Check sheet for the modelled part. Datum: model origin and axes. Units: mm. A direction names the side the tool comes from. Coordinates: 2 decimals unless noted, no trailing zeros. Loops run counter-clockwise (first coordinate to the right, second up) from the corner with the lowest first, then second, coordinate; pieces in that order, holes last. Notation, with made-up numbers: M -28,-23.75 L -21,-23.75 A34 cw -21,11.25 Z; hole C -14,-15.5 d8. An arc over 180 degrees is marked long. Return JSON: item names as keys, results as strings.
from build123d import *

# Parameters (mm, degrees)
SKETCH1_R           = 9.5
SKETCH1_R_2         = 3
BOSS_EXTRUDE1_DEPTH = 6


with BuildPart() as part:
    # Sketch1 → Boss-Extrude1 (new body)
    with BuildSketch(Plane(origin=(0, 0, 0), x_dir=(1, 0, 0), z_dir=(0, 1, 0))):
        Circle(SKETCH1_R)
        Circle(SKETCH1_R_2, mode=Mode.SUBTRACT)
    extrude(amount=BOSS_EXTRUDE1_DEPTH)

    # Sketch2 → Cut-Revolve1 (revolve, cut)
    with BuildSketch(Plane.XY):
        Polygon((-3.75, 6), (-4.75, 5.5), (-7.75, 5.5), (-8.75, 6), align=None)
        Polygon((-8.75, 0), (-3.75, 0), (-4.75, 0.5), (-7.75, 0.5), align=None)
    revolve(axis=Axis((0, 6, 0), (0, -1, 0)), mode=Mode.SUBTRACT)


solid = part.part
1) Section check A-A on x = 0. Record the cut outline in (y, z).
Answers:
{"outline": "M 0,-9.5 L 6,-9.5 L 6,-8.75 L 5.5,-7.75 L 5.5,-4.75 L 6,-3.75 L 6,-3 L 0,-3 L 0,-3.75 L 0.5,-4.75 L 0.5,-7.75 L 0,-8.75 Z; M 0,3 L 6,3 L 6,3.75 L 5.5,4.75 L 5.5,7.75 L 6,8.75 L 6,9.5 L 0,9.5 L 0,8.75 L 0.5,7.75 L 0.5,4.75 L 0,3.75 Z"}
2) Draft check along X on faces 4 (the face through (4.38, 2.96, 8.43)), 5 (the face through (-3, 3, 0)), 6 (the face through (1, 0, -3)). Enter one of: +X half, -X half, draft (parallel to the pull), parting line (faces both ways), or undercut.
Answers:
{"face 4": "parting line", "face 5": "undercut", "face 6": "draft"}
3) Scan lines: line 1 along X through (y, z) = (1.95, 0); line 2 along X through (y, z) = (2.15, 2.25). Record each from-to range of solid material in increasing order. Write a range as [from, to].
Answers:
{"line 1": "[-9.5, -3], [3, 9.5]", "line 2": "[-9.23, -1.98], [1.98, 9.23]"}
4) Go/stop test with flat-tipped pins: pin 1 Ø2 at (y, z) = (4, 4) entering from +X; pin 2 Ø2 at (y, z) = (4.5, -3.5) entering from -X; pin 3 Ø5 at (x, z) = (0, 0) entering from -Y; pin 4 Ø4 at (x, z) = (6, 3) entering from +Y. Record where each tip stops, or that it passes through.
Answers:
{"pin 1": "x = 9.01", "pin 2": "x = -9.17", "pin 3": "through", "pin 4": "y = 5.98"}
5) Section check B-B on z = 0. Record the cut outline in (x, y).
Answers:
{"outline": "M -9.5,0 L -8.75,0 L -7.75,0.5 L -4.75,0.5 L -3.75,0 L -3,0 L -3,6 L -3.75,6 L -4.75,5.5 L -7.75,5.5 L -8.75,6 L -9.5,6 Z; M 3,0 L 3.75,0 L 4.75,0.5 L 7.75,0.5 L 8.75,0 L 9.5,0 L 9.5,6 L 8.75,6 L 7.75,5.5 L 4.75,5.5 L 3.75,6 L 3,6 Z"}
6) Section check C-C on y = 2.25. Record the cut outline in (x, z).
Answers:
{"outline": "C 0,0 d19; hole C 0,0 d6"}
7) Set-up check for faces 1 (the face through (-4, 0.5, 3)), 2 (the face through (-4, 5.5, 3)), 3 (the face through (4, 6, 8)): record each of +Z, -Z, +X, -X, +Y, -Y from which the full face is reachable in a straight line by a thin tool's end or side.
Answers:
{"face 1": "-Y", "face 2": "+Y", "face 3": "+Z, -Z, +X, -X, +Y"}
